The drawing under review shows one solid part. Ordinate dimensions are in mm from its lowest x, y, z. Give positions to 0.01 mm unless a question says otherwise; leave off trailing zeros. Write each loop counter-clockwise with the first axis right and the second up, starting at its lowest first coordinate (ties: lowest second). Pieces come first, ordered by that corner, then holes. Notation, with made-up numbers: M 36,52.25 L 56,52.25 A5 cw 56,59.25 Z; hole C 84,47 d7. An arc over 180 degrees is marked long. Answer as a JSON object with one key per item and string values. Group by question number.
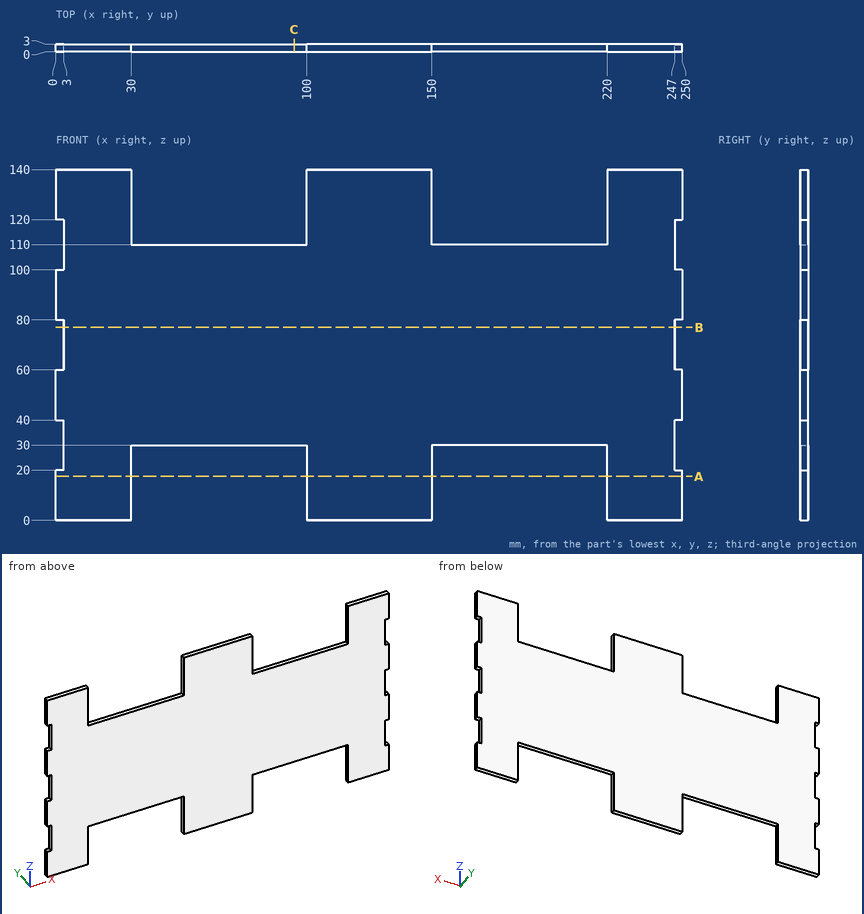
Item 1: To check wall thickness, follow probe 1 along X at (y, z) = (2.15, 122.5); probe 2 along X at (y, z) = (0.25, 111); probe 3 along Z at (x, y) = (210.5, 2.8). State the ranges of each line that lie inside material, in increasing order.
Item 2: Consider section A-A (z = 17.5). Give the boundary of the cut face in (x, y), plus the area to 3 significant figures.
Item 3: Insertion check: P1, Ø1.5, axis at y = 2, z = 37.5, coming from the -X side; P2, Ø1.5, axis at x = 248, y = 1.5, coming from the -Z side; P3, Ø1.5, axis at x = 168.5, y = 1.5, coming from the +Z side; P4, Ø1.5, axis at y = 2, z = 21, coming from the +X side. Each pin has a flat end and moves straight along its axis. Give the tip position at first contact, or say it passes through.
Item 4: Consider section B-B (z = 77). Give the boundary of the cut face in (x, y), plus the area to 3 significant figures.
Item 5: Consider section C-C (x = 95). Give the boundary of the cut face in (y, z).
Result set:
{
 "1": {"probe 1": "x = 0 to 30, 100 to 150, 220 to 250", "probe 2": "x = 3 to 30, 100 to 150, 220 to 247", "probe 3": "z = 30 to 110"},
 "2": {"outline": "M 0,0 L 30,0 L 30,3 L 0,3 Z; M 100,0 L 150,0 L 150,3 L 100,3 Z; M 220,0 L 250,0 L 250,3 L 220,3 Z", "area": "330 mm^2"},
 "3": {"P1": "stops at x = 3", "P2": "stops at z = 0", "P3": "stops at z = 110", "P4": "stops at x = 247"},
 "4": {"outline": "M 3,0 L 247,0 L 247,3 L 3,3 Z", "area": "732 mm^2"},
 "5": {"outline": "M 0,30 L 3,30 L 3,110 L 0,110 Z"}
}
